Answer from the drawing. Dimensions are ordinates in mm from the lowest x, y and z of the part. A direction names the side the tool comes from. Coordinates: 2 decimals unless noted, no trailing zeros. Loops run counter-clockwise (first coordinate to the right, second up) from the corner with the lowest first, then second, coordinate; pieces in that order, holes last. Notation, with made-up numbers: M -38,3 L -13,3 A20 ccw -13,35 Z; hole C 5.5,87.25 d6. An arc over 180 degrees is marked long. Put each result on its own line as item: value.
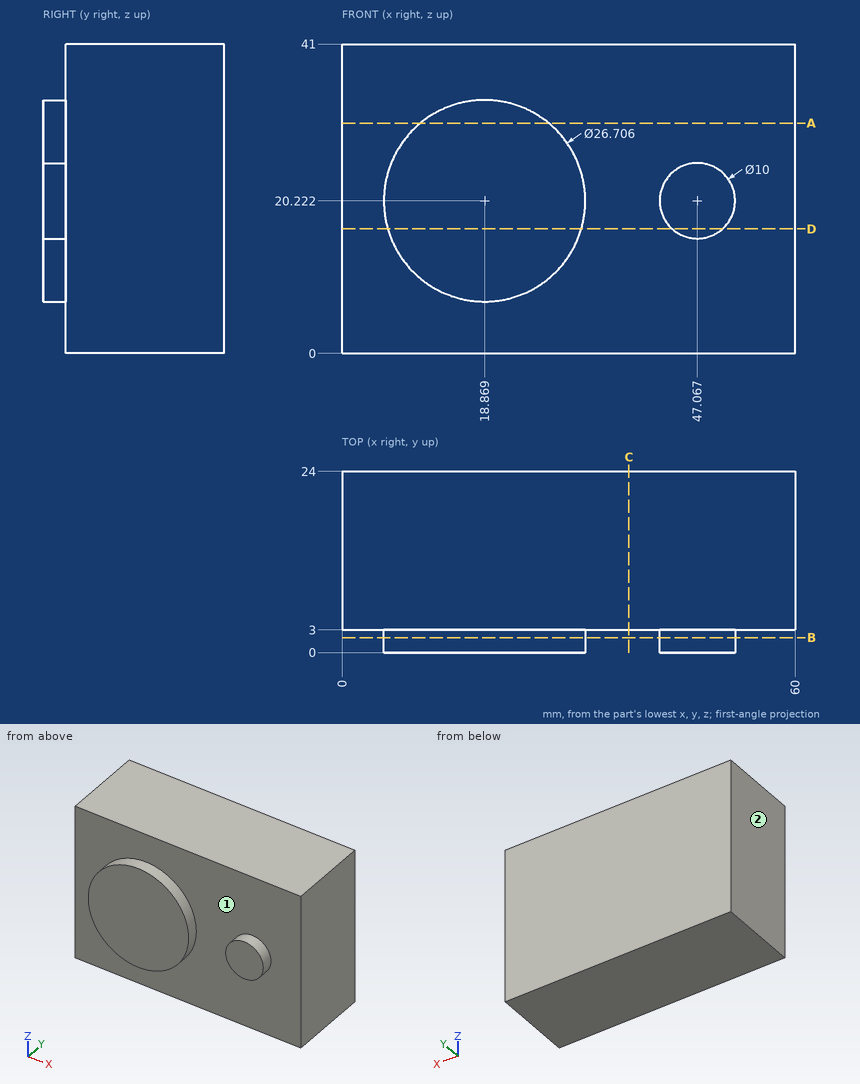
1) Find section D-D, the plane z = 16.5. Write down the section's boundary in (x, y) (1 decimal), plus the area to 3 significant figures.
Answer list:
outline: M 0,3 L 6,3 L 6,0 L 31.7,0 L 31.7,3 L 43.7,3 L 43.7,0 L 50.4,0 L 50.4,3 L 60,3 L 60,24 L 0,24 Z
area: 1,360 mm^2
2) Which of the six approach directions +Z, -Z, +X, -X, +Y, -Y give full straight-line access (tool end or side, diameter ignored) to the marked faces 1 and 2?
Answer list:
face 1: -Y
face 2: +Z, -Z, -X, +Y, -Y
3) Straight lines are drawn through the part: line 1 (Y direction, x = 42, z = 34.5); line 2 (Z direction, x = 47, y = 2); line 3 (X direction, y = 1, z = 12.5) (1 decimal). For each, find the intervals that lie inside material, in ascending order. Write a range as [from, to].
Answer list:
line 1: y = [3, 24]
line 2: z = [15.22, 25.22]
line 3: x = [8, 29.8]
4) Given pin 1 Ø2 at (x, z) = (42, 31.5) entering from -Y, flat-ended and moving along its own axis, determine where the tip first touches the part or whether it passes through.
Answer list:
pin 1: stops at y = 3
5) Find section B-B, the plane y = 2. Write down the section's boundary in (x, z), plus the area to 3 significant figures.
Answer list:
outline: C 18.87,20.22 d26.71; C 47.07,20.22 d10
area: 639 mm^2
6) Find section A-A, the plane z = 30.5. Write down the section's boundary in (x, y) (1 decimal), plus the area to 3 significant figures.
Answer list:
outline: M 0,3 L 10.3,3 L 10.3,0 L 27.4,0 L 27.4,3 L 60,3 L 60,24 L 0,24 Z
area: 1,310 mm^2
7) Find section C-C, the plane x = 38. Write down the section's boundary in (y, z), plus the area to 3 significant figures.
Answer list:
outline: M 3,0 L 24,0 L 24,41 L 3,41 Z
area: 861 mm^2
